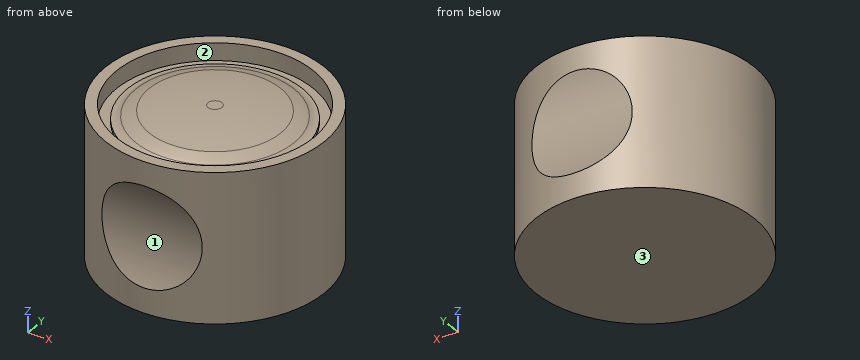
from build123d import *

# Parameters (mm, degrees)
F2_R     = 12.5
F2_R_2   = 10
F3_DEPTH = 15
F4_R     = 12.5
F4_R_2   = 11.25
F5_DEPTH = 2
F8_DEPTH = 50


with BuildPart() as f1:
    # F0 (on Front) → F1 (revolve)
    with BuildSketch(Plane.XZ):
        with BuildLine():
            Line((4.9800029832, -0.7875902065), (4.9800029832, -0.3815757062))
            Line((4.9800029832, -0.3815757062), (4.9800029832, 1.1184242938))
            Line((4.9800029832, 1.1184242938), (4.1800029832, 1.1184242938))
            ThreePointArc((4.1800029832, 1.1184242938), (0.8118554552, 0.9601863869), (-2.5266210559, 0.4868666314))
            ThreePointArc((-2.5266210559, 0.4868666314), (-3.3020091302, 0.2364900314), (-4.0513253894, -0.083572855))
            ThreePointArc((-4.0513253894, -0.083572855), (-4.5132598016, -0.3053910404), (-5.0199970168, -0.3815757062))
            Line((-5.0199970168, -0.3815757062), (-5.0199970168, -0.7875902065))
            Line((-5.0199970168, -0.7875902065), (4.9800029832, -0.7875902065))
        make_face()
    revolve(axis=Axis((4.9800029832, 0, 0.3684242938), (0, 0, 1)))

    # F2 (on face) → F3 (join)
    with BuildSketch(Plane(origin=(0, 0, -0.7875902065), x_dir=(1, 0, 0), z_dir=(0, 0, -1))):
        with Locations((4.9800029832, 0)):
            Circle(F2_R)
        with Locations((4.9800029832, 0)):
            Circle(F2_R_2, mode=Mode.SUBTRACT)
        with Locations((4.9800029832, 0)):
            Circle(F2_R_2)
    extrude(amount=F3_DEPTH)

    # F4 (on face) → F5 (join)
    with BuildSketch(Plane.XY.offset(-0.7875902065)):
        with Locations((4.9800029832, 0)):
            Circle(F4_R)
        with Locations((4.9800029832, 0)):
            Circle(F4_R_2, mode=Mode.SUBTRACT)
    extrude(amount=F5_DEPTH)

    # F7 (on offset) → F8 (cut)
    with BuildSketch(Plane.YZ.offset(17.3)):
        with BuildLine():
            Line((-13.25, -0.238639344), (-13.25, -14.238639344))
            ThreePointArc((-13.25, -14.238639344), (-11.1241774834, -7.238639344), (-13.25, -0.238639344))
        make_face()
        with BuildLine():
            ThreePointArc((13.25, -0.238639344), (11.1241774834, -7.238639344), (13.25, -14.238639344))
            Line((13.25, -14.238639344), (13.25, -0.238639344))
        make_face()
    extrude(amount=-F8_DEPTH, mode=Mode.SUBTRACT)


solid = f1.part
Input: part model. Units: mm. Frame: model coordinates. Face numbers are marked on the shaded views. Coordinates: 2 decimals unless noted, no trailing zeros. Loops run counter-clockwise (first coordinate to the right, second up) from the corner with the lowest first, then second, coordinate; pieces in that order, holes last. Notation, with made-up numbers: (69, -15) -> (122, -15) arc R19 ccw to (122, 12) -> close; hole circle Ø8 at (85, -23). An arc over 180 degrees is marked (long way). Write item = value, one per line. Start each with the question number.
Item 1: Cut plane A-A, the plane z = -3.5. Return loops of the section in (x, y), plus the area to 3 significant figures.
Item 2: Material intervals for line 1 (Y direction, x = 7.5, z = -7.5); line 2 (X direction, y = -7.5, z = -12.5); line 3 (Z direction, x = 5.5, y = -11), sorted ascending.
Item 3: Mould query, pull axis Y, two halves, no side actions, for the marked faces 1, 2 and 3. Classes: pulls with the +Y half, pulls with the -Y half, needs draft (parallel to the pull), parting line crosses it, or undercut.
Item 4: First-contact query: P1, Ø4, axis at x = 4, z = -4, coming from the +Y side; P2, Ø8, axis at x = -1, z = -2, coming from the -Y side; P3, Ø10, axis at x = 14, z = -5.5, coming from the +Y side. Flat tips, straight axial feed; report the tip coordinate or a pass-through.
Item 5: Cut plane B-B, the plane z = -6. Return loops of the section in (x, y).
Ans:
q1.outline = (0.56, -11.69) -> (9.4, -11.69) arc R12.5 ccw to (9.4, 11.69) -> (0.56, 11.69) arc R12.5 ccw to start
q1.area = 481 mm²
q2.line_1 = -11.13 to 11.13
q2.line_2 = -5.02 to 14.98
q2.line_3 = -15.79 to -0.79
q3.face_1 = pulls with the -Y half
q3.face_2 = undercut
q3.face_3 = needs draft
q4.P1 = 12.27
q4.P2 = -12.34
q4.P3 = 11.69
q5.outline = (-0.6, -11.19) -> (10.56, -11.19) arc R12.5 ccw to (10.56, 11.19) -> (-0.6, 11.19) arc R12.5 ccw to start
